Part model, mm, in its own coordinate system. A direction names the side the tool comes from. Give positions to 0.01 mm unless a question says otherwise; leave off trailing zeros. Write each loop counter-clockwise with the first axis right and the second up, starting at its lowest first coordinate (ties: lowest second). Pieces come first, ordered by that corner, then holes.
Autodesk Inventor part; units mm, degrees
ref_plane "YZ Plane" through (0, 0, 0) normal (1, 0, 0) x (0, 1, 0)
ref_plane "XZ Plane" through (0, 0, 0) normal (0, 1, 0) x (-1, 0, 0)
ref_plane "XY Plane" through (0, 0, 0) normal (0, 0, 1) x (1, 0, 0)
sketch "Sketch1" plane through (0, 0, 0) normal (1, 0, 0) x (0, 1, 0)
  line L0 (0, 0) -> (50.8, 0)
  line L1 (0, 138.1125) -> (26.719, 138.1125)
  line L2 (0, 138.1125) -> (0, 169.8625)
  line L3 (0, 169.8625) -> (3.175, 169.8625)
  line L4 (3.175, 169.8625) -> (3.175, 141.2875)
  line L5 (3.175, 141.2875) -> (22.9489, 141.2875)
  line L6 (60.325, 141.2875) -> (60.325, 179.3875)
  line L7 (60.325, 179.3875) -> (63.5, 179.3875)
  line L8 (63.5, 179.3875) -> (63.5, 138.1125)
  line L9 (35.6489, 138.1125) -> (26.719, 138.1125)
  line L10 (29.2989, 139.7) -> (22.9489, 139.7)
  line L11 (22.9489, 139.7) -> (22.9489, 141.2875)
  line L12 (29.2989, 139.7) -> (35.6489, 139.7)
  line L13 (35.6489, 139.7) -> (35.6489, 138.1125)
  line L14 (29.2989, 166.1379) -> (29.2989, 141.2875)
  line L15 (29.2989, 138.1125) -> (29.2989, 120.1049)
  point P0 (62.1333, 179.3875)
  point P1 (1.5875, 169.8625)
  dimension "d0" = 50.8
  dimension "d1" = 138.1125
  dimension "d2" = 31.75
  dimension "d3" = 3.175
  dimension "d4" = 3.175
  dimension "d5" = 57.15
  dimension "d6" = 38.1
  dimension "d7" = 3.175
  dimension "d13" = 26.1239
  dimension "d14" = 1.5875
  dimension "d15" = 6.35
  dimension "d16" = 6.35
revolve "Revolution1" add sketch "Sketch1" angle 360 about axis through (0, 0, 0) along (0, 1, 0)
ref_plane "Work Plane2" through (0, 1.5875, 169.8625) normal (0, 0, 1) x (1, 0, 0)
sketch "Sketch3" plane through (0, 1.5875, 169.8625) normal (0, 0, 1) x (1, 0, 0)
  arc A0 (-6.3749, 27.6865) -> (6.3749, 27.6865) centre (0, 27.6865) ccw
  line L0 (138.1125, 34.0614) -> (-138.1125, 34.0614)
  line L1 (-6.3749, 27.6865) -> (-6.3749, 34.0614)
  line L2 (6.3749, 27.6865) -> (6.3749, 34.0614)
  point P0 (0, -1.5875)
  point P1 (0, 17.4621)
extrude "Extrusion2" cut sketch "Sketch3" against normal through all
properties part number "Layer2_Bottom"
1) Saw through at C-C (y = 14). Write the cut outline in (x, z) (1 decimal).
Check result:
outline: circle Ø282.6 at (0, 0); hole circle Ø276.2 at (0, 0)
2) Saw through at B-B (z = -131.5). Write the cut outline in (x, y) (3 decimals).
Check result:
outline: (-107.522, 0) - (-42.223, 0) - (-42.223, 35.649) - (-47.158, 35.649) - (-47.158, 22.949) - (-51.671, 22.949) - (-51.671, 3.175) - (-107.522, 3.175) - close; (42.223, 0) - (107.522, 0) - (107.522, 3.175) - (51.671, 3.175) - (51.671, 22.949) - (47.158, 22.949) - (47.158, 35.649) - (42.223, 35.649) - close
3) Flat gauge pins, fed straight in: P1, Ø6, axis at x = -113, y = 14, coming from the -Z side; P2, Ø8, axis at y = 24, z = 92.5, coming from the -X side; P3, Ø12, axis at x = -22.5, y = 8.5, coming from the +Z side. Where does each tip first touch, or does it go through?
Check result:
P1: stops at z = -88.67
P2: stops at x = -110.02
P3: stops at z = 168.71
4) Drill centre lines: L1, parallel to Z at x = 0, y = 7; L2, parallel to X at y = 23.5, z = 0. Where is each one in solid material? Low to high.
Check result:
L1: z = -141.29 to -138.11, 138.11 to 141.29
L2: x = -139.7 to -138.11, 138.11 to 139.7
5) Saw through at A-A (x = -47). Write the cut outline in (y, z) (3 decimals), and give its area (3 significant figures).
Check result:
outline: (0, -163.231) - (3.175, -163.231) - (3.175, -133.241) - (22.949, -133.241) - (22.949, -131.556) - (35.649, -131.556) - (35.649, -129.869) - (0, -129.869) - close; (0, 129.869) - (35.649, 129.869) - (35.649, 131.556) - (22.949, 131.556) - (22.949, 133.241) - (3.175, 133.241) - (3.175, 163.231) - (0, 163.231) - close
area: 388 mm2
6) 3-axis set-ups, long thin cutter, end or side, ignore diameter. For faces 1 (the cylindrical face through (119.13, 13.2, 75.96)), 2 (the flat face through (139, 0, -1)), 3 (the cylindrical face through (139.666, 29.21, -3.061)), 4 (the cylindrical face through (-165.823, 1.61, -36.823)), 5 (the cylindrical face through (-139.666, 29.21, 3.061)): which of +Z, -Z, +X, -X, +Y, -Y reach the whole face in a straight line?
Check result:
face 1: +Y
face 2: +Z, -Z, +X, -X, -Y
face 3: +X, +Y
face 4: +Y, -Y
face 5: -X, +Y
